Check sheet for the modelled part. Datum: model origin and axes. Units: mm. A direction names the side the tool comes from. Coordinates: 2 decimals unless noted, no trailing zeros. Order: outer loops, then holes, each group sorted by start corner. A loop starts at its lowest first (then second) coordinate and runs counter-clockwise, first axis right, second up.
1. Gauge pin test, flat ends, axial feed: pin 1 Ø1.6 at (x, y) = (24.5, 0) entering from -Z; pin 2 Ø3.5 at (x, y) = (-13, 2) entering from +Z; pin 3 Ø2.5 at (y, z) = (1.5, 3.5) entering from +X. Record the tip position at first contact, or that the pin passes through.
2. Cross-section at C-C (z = -21.5). Enter the section's corners in (x, y).
3. Cross-section at D-D (x = 18). Enter the section's corners in (y, z), then the cut area to 3 significant figures.
4. Cross-section at A-A (y = 1). Enter the section's corners in (x, z).
5. Cross-section at B-B (x = -5). Enter the section's corners in (y, z), then the cut area to 3 significant figures.
6. Set-up check for faces 1 (the flat face through (-22, 0, -110)), 2 (the flat face through (13, 1, 0)), 3 (the flat face through (-13, 1, 0)), 4 (the flat face through (0, 0, -29)): record each of +Z, -Z, +X, -X, +Y, -Y from which the full face is reachable in a straight line by a thin tool's end or side.
7. Thickness scan on line 1 (Z direction, x = -7, y = -2.05); line 2 (Z direction, x = 22.5, y = -1.4); line 3 (Y direction, x = -4, z = -6.5). Record the ranges inside material, lowest first.
```python
from build123d import *

# Parameters (mm, degrees)
BOSS_EXTRUDE1_DEPTH = 3
BOSS_EXTRUDE2_DEPTH = 3


with BuildPart() as part:
    # Sketch1 → Boss-Extrude1 (new body)
    with BuildSketch(Plane(origin=(0, 0, 0), x_dir=(1, 0, 0), z_dir=(0, 1, 0))):
        Polygon((-22, 64), (-16.5, 0), (-10, 0), (-10, -6.5), (10, -6.5), (10, 0), (16.5, 0), (23.1, 64), (27.3, 64), (27.3, 108.3), (22, 108.3), (22, 111.6), (-22, 111.6), (-22, 108.3), (-27.3, 108.3), (-27.3, 64), align=None)
    extrude(amount=BOSS_EXTRUDE1_DEPTH)

    # Sketch3 → Boss-Extrude2 (add)
    with BuildSketch(Plane.XZ):
        Polygon((-27.3, -64), (-27.3, -108.3), (-22, -108.3), (-22, -111.6), (22, -111.6), (22, -108.3), (27.3, -108.3), (27.3, -64), (23.1, -64), (-22, -64), align=None)
    extrude(amount=BOSS_EXTRUDE2_DEPTH)


solid = part.part
```
Data:
1. pin 1: stops at z = -108.3
1. pin 2: stops at z = 0
1. pin 3: stops at x = 10
2. outline: (-18.35, 0) - (18.72, 0) - (18.72, 3) - (-18.35, 3) - close
3. outline: (-3, -111.6) - (3, -111.6) - (3, -14.55) - (0, -14.55) - (0, -64) - (-3, -64) - close
3. area: 434 mm2
4. outline: (-27.3, -108.3) - (-22, -108.3) - (-22, -111.6) - (22, -111.6) - (22, -108.3) - (27.3, -108.3) - (27.3, -64) - (23.1, -64) - (16.5, 0) - (10, 0) - (10, 6.5) - (-10, 6.5) - (-10, 0) - (-16.5, 0) - (-22, -64) - (-27.3, -64) - close
5. outline: (-3, -111.6) - (3, -111.6) - (3, 6.5) - (0, 6.5) - (0, -64) - (-3, -64) - close
5. area: 497 mm2
6. face 1: -Z, -X, +Y, -Y
6. face 2: +Z, +X, +Y, -Y
6. face 3: +Z, -X, +Y, -Y
6. face 4: +Z, +X, -X, -Y
7. line 1: z = -111.6 to -64
7. line 2: z = -108.3 to -64
7. line 3: y = 0 to 3
